Work out the finished part from the listing and answer in its coordinate system (mm). A direction names the side the tool comes from. Round coordinates to 2 decimals unless told otherwise and drop trailing zeros. Loops run counter-clockwise (first coordinate to the right, second up) from the corner with the lowest first, then second, coordinate; pieces in that order, holes last.
```python
from build123d import *

# Parameters (mm, degrees)
F0_W     = 762
F0_H     = 25.4
F1_DEPTH = 25.4
F2_W     = 19.05
F2_H     = 44.45
F3_DEPTH = 762.001
F4_R     = 2.4892
F5_DEPTH = 50.801


with BuildPart() as f1:
    # F0 (on Top) → F1 (new body, symmetric)
    with BuildSketch(Plane.XY):
        Rectangle(F0_W, F0_H)
    extrude(amount=F1_DEPTH, both=True)

    # F2 (on face) → F3 (cut, through all)
    with BuildSketch(Plane.YZ.offset(381)):
        Rectangle(F2_W, F2_H)
    extrude(amount=-F3_DEPTH, mode=Mode.SUBTRACT)

    # F4 (on face) → F5 (cut, through all)
    with BuildSketch(Plane.XY.offset(25.4)):
        with Locations((-368.3, 0)):
            Circle(F4_R)
        with Locations((-342.9, 0)):
            Circle(F4_R)
        with Locations((-317.5, 0)):
            Circle(F4_R)
        with Locations((-292.1, 0)):
            Circle(F4_R)
        with Locations((-266.7, 0)):
            Circle(F4_R)
        with Locations((-241.3, 0)):
            Circle(F4_R)
        with Locations((-215.9, 0)):
            Circle(F4_R)
        with Locations((-190.5, 0)):
            Circle(F4_R)
        with Locations((-165.1, 0)):
            Circle(F4_R)
        with Locations((-139.7, 0)):
            Circle(F4_R)
        with Locations((-114.3, 0)):
            Circle(F4_R)
        with Locations((-88.9, 0)):
            Circle(F4_R)
        with Locations((-63.5, 0)):
            Circle(F4_R)
        with Locations((-38.1, 0)):
            Circle(F4_R)
        with Locations((-12.7, 0)):
            Circle(F4_R)
        with Locations((12.7, 0)):
            Circle(F4_R)
        with Locations((38.1, 0)):
            Circle(F4_R)
        with Locations((63.5, 0)):
            Circle(F4_R)
        with Locations((88.9, 0)):
            Circle(F4_R)
        with Locations((114.3, 0)):
            Circle(F4_R)
        with Locations((139.7, 0)):
            Circle(F4_R)
        with Locations((165.1, 0)):
            Circle(F4_R)
        with Locations((190.5, 0)):
            Circle(F4_R)
        with Locations((215.9, 0)):
            Circle(F4_R)
        with Locations((241.3, 0)):
            Circle(F4_R)
        with Locations((266.7, 0)):
            Circle(F4_R)
        with Locations((292.1, 0)):
            Circle(F4_R)
        with Locations((317.5, 0)):
            Circle(F4_R)
        with Locations((342.9, 0)):
            Circle(F4_R)
        with Locations((368.3, 0)):
            Circle(F4_R)
    extrude(amount=-F5_DEPTH, mode=Mode.SUBTRACT)


solid = f1.part
```
1. Find section B-B (x = 303). Write down the section's boundary in (y, z) (3 decimals), then the cut area to 3 significant figures.
Answer key:
outline: (-12.7, -25.4) - (12.7, -25.4) - (12.7, 25.4) - (-12.7, 25.4) - close; hole (-9.525, -22.225) - (9.525, -22.225) - (9.525, 22.225) - (-9.525, 22.225) - close
area: 444 mm2
2. Determine the mould class of faces 1 (the face through (-5, 12.7, 0)), 2 (the face through (-381, -10, -2)), 3 (the face through (5, 0, -22.225)) for opening direction Y: +Y half, -Y half, draft (parallel to the pull), parting line (faces both ways), or undercut.
Answer key:
face 1: +Y half
face 2: draft
face 3: undercut
3. Consider probe 1 along Y at (x, z) = (-145.5, -4.5) (3 decimals); probe 2 along Z at (x, y) = (-314.5, 0.75) (3 decimals); probe 3 along Y at (x, z) = (-88.9, -23.1). Determine where each line is inside the solid, lowest interval first.
Answer key:
probe 1: y = -12.7 to -9.525, 9.525 to 12.7
probe 2: z = -25.4 to -22.225, 22.225 to 25.4
probe 3: y = -12.7 to -2.49, 2.49 to 12.7
4. Which of the six approach directions +Z, -Z, +X, -X, +Y, -Y give full straight-line access (tool end or side, diameter ignored) to faces 4 (the face through (5, 0, 22.225)), 5 (the face through (-5, -12.7, 0))?
Answer key:
face 4: +X, -X
face 5: +Z, -Z, +X, -X, -Y
5. Given pin 1 (10 mm diameter, centred on y = 4, z = 13, fed in from +X), flat-ended and moving along its own axis, determine where the tip first touches the part or whether it passes through.
Answer key:
pin 1: passes through
6. Find section A-A (z = -10). Write down the section's boundary in (x, y) (3 decimals), then the cut area to 3 significant figures.
Answer key:
outline: (-381, -12.7) - (381, -12.7) - (381, -9.525) - (-381, -9.525) - close; (-381, 9.525) - (381, 9.525) - (381, 12.7) - (-381, 12.7) - close
area: 4,840 mm2
